```python
from build123d import *

# Parameters (mm, degrees)
FILETE1_R             = 1
FILETE2_R             = 2
ESBO_O2_R             = 2.5
CORTE_EXTRUS_O1_DEPTH = 74.773875806


with BuildPart() as part:
    # Esboço1 → Revolução1 (revolve)
    with BuildSketch(Plane.XY, mode=Mode.PRIVATE) as revolu_o1_sk:
        with BuildLine():
            Line((52, 4.149133087), (52, -0.850866913))
            ThreePointArc((52, -0.850866913), (47.161295888, -1.704708432), (42.5, -0.150866913))
            Line((42.5, -0.150866913), (40.5, -0.150866913))
            Line((40.5, -0.150866913), (40.5, 1.149133087))
            Line((40.5, 1.149133087), (42.5, 1.149133087))
            Line((42.5, 1.149133087), (42.5, 4.149133087))
            Line((42.5, 4.149133087), (52, 4.149133087))
        make_face()
    revolve(revolu_o1_sk.sketch.rotate(Axis((0, -12.642652583, 0), (0, 1, 0)), 90), axis=Axis((0, -12.642652583, 0), (0, 1, 0)))

    # Filete1
    filete1_edges = [part.edges().sort_by_distance(p)[0] for p in [
        (0, 1.149133087, 42.5),
    ]]
    fillet(filete1_edges, radius=FILETE1_R)

    # Filete2
    filete2_edges = [part.edges().sort_by_distance(p)[0] for p in [
        (0, -0.150866913, 42.5),
    ]]
    fillet(filete2_edges, radius=FILETE2_R)

    # Esboço2 → Corte-extrusão1 (cut, through all)
    with BuildSketch(Plane(origin=(0, 4.149133087, 0), x_dir=(1, 0, 0), z_dir=(0, 1, 0))):
        with Locations(Location((-46, 0, 0), (0, 0, 270))):
            Circle(ESBO_O2_R)
        with Locations(Location((23, 39.837168574, 0), (0, 0, 270))):
            Circle(ESBO_O2_R)
        with Locations(Location((23, -39.837168574, 0), (0, 0, 270))):
            Circle(ESBO_O2_R)
    extrude(amount=-CORTE_EXTRUS_O1_DEPTH, mode=Mode.SUBTRACT)


solid = part.part
```
Work out the finished part from the listing and answer in its coordinate system (mm). A direction names the side the tool comes from. Round coordinates to 2 decimals unless told otherwise and drop trailing zeros.
Q1. A tool of negligible diameter and unlimited length cuts with its end or side. For faces 4 (the cylindrical face through (-48.44, 1.25, -0.54)), 5 (the flat face through (40, 1.149, 9)), 6 (the flat face through (41.6, -0.151, 0.2)), from which of +Z, -Z, +X, -X, +Y, -Y can it reach the whole face along a straight path? Write none if from no direction.
Solution:
face 4: +Y, -Y
face 5: +Y
face 6: -Y
Q2. A cutting plane is placed at A-A, the plane x = 23. Count the separate pieces of the cut face and the enclosed holes in it, then the cut area to 3 significant figures.
Solution:
separate pieces: 4
enclosed holes: 0
area: 69.7 mm2
Q3. Find the intervals of material crossed by line 1 along Y through (x, z) = (40, -10); line 2 along Z through (x, y) = (-35.5, 2.65); line 3 along X through (y, z) = (1.85, 33.5), in increasing order.
Solution:
line 1: y = -0.15 to 1.15
line 2: z = -38 to -23.37, 23.37 to 38
line 3: x = -39.77 to -26.08, 26.08 to 39.77
Q4. The mould has two halves that part along Z. Classify faces 1 (the flat face through (4, 4.149, -43)), 2 (the cylindrical face through (24.69, 1.25, -41.68)), 3 (the cylindrical face through (31.641, 1.614, 41.265)): pulls with the +Z half, pulls with the -Z half, needs draft (parallel to the pull), parting line crosses it, or undercut.
Solution:
face 1: needs draft
face 2: undercut
face 3: parting line crosses it
Q5. Given pin 1 Ø8 at (x, z) = (-6, 35.5) entering from +Y; pin 2 Ø2 at (y, z) = (0.5, 39) entering from +X; pin 3 Ø3 at (x, y) = (30, 1.5) entering from +Z; pin 4 Ø1 at (x, y) = (19.5, 2.5) entering from -Z, each flat-ended and moving along its own axis, determine where each tip first touches the part or whether it passes through.
Solution:
pin 1: passes through
pin 2: stops at x = 35.5
pin 3: stops at z = 43.49
pin 4: stops at z = -48.4
